Design review of the part shown in the three views and the two pictorial views. Dimensions are in mm from the part's minimum x, y and z. A direction names the side the tool comes from. Coordinates: 2 decimals unless noted, no trailing zeros. Order: outer loops, then holes, each group sorted by start corner. A loop starts at its lowest first (then second) coordinate and runs counter-clockwise, first axis right, second up. Notation, with made-up numbers: (-19.75, 1.5) - (27.25, 1.5) arc R31 cw to (27.25, 30.5) - close; hole circle Ø2 at (64.5, 84). An arc over 180 degrees is marked (long way). One line per item, written item: value. Start each with the question number.
(1) Clearance check with a flat-ended pin moving along its axis: pin 1 (2 mm diameter, centred on x = 5.5, z = 3.5, fed in from -Y). State where the tip first meets the part, or that it passes through.
(2) To check wall thickness, follow line 1 along Z through (x, y) = (0.5, 0.5); line 2 along Y through (x, z) = (5.5, 6.75); line 3 along Z through (x, y) = (4.25, 14). State the ranges of each line that lie inside material, in increasing order.
(3) For the marked faces 1 and 2, list the 3-axis set-ups (+Z, -Z, +X, -X, +Y, -Y) from which the entire face can be reached by the end or side of a thin tool; tool diameter is ignored.
(4) Mouldability with a two-part tool opening along Z and no side actions: class the marked faces 3, 4, 5 and 6 as released by +Z, released by -Z, zero draft, split by the parting line, or undercut.
(5) Consider section A-A on y = 8.25. Write out the cut boundary in (x, z), then the cut area to 3 significant figures.
(6) Consider section C-C on x = 10.75. Write out the cut boundary in (y, z).
(7) Consider section D-D on y = 4. Write out the cut boundary in (x, z).
(8) Consider section B-B on z = 5. Write out the cut boundary in (x, y).
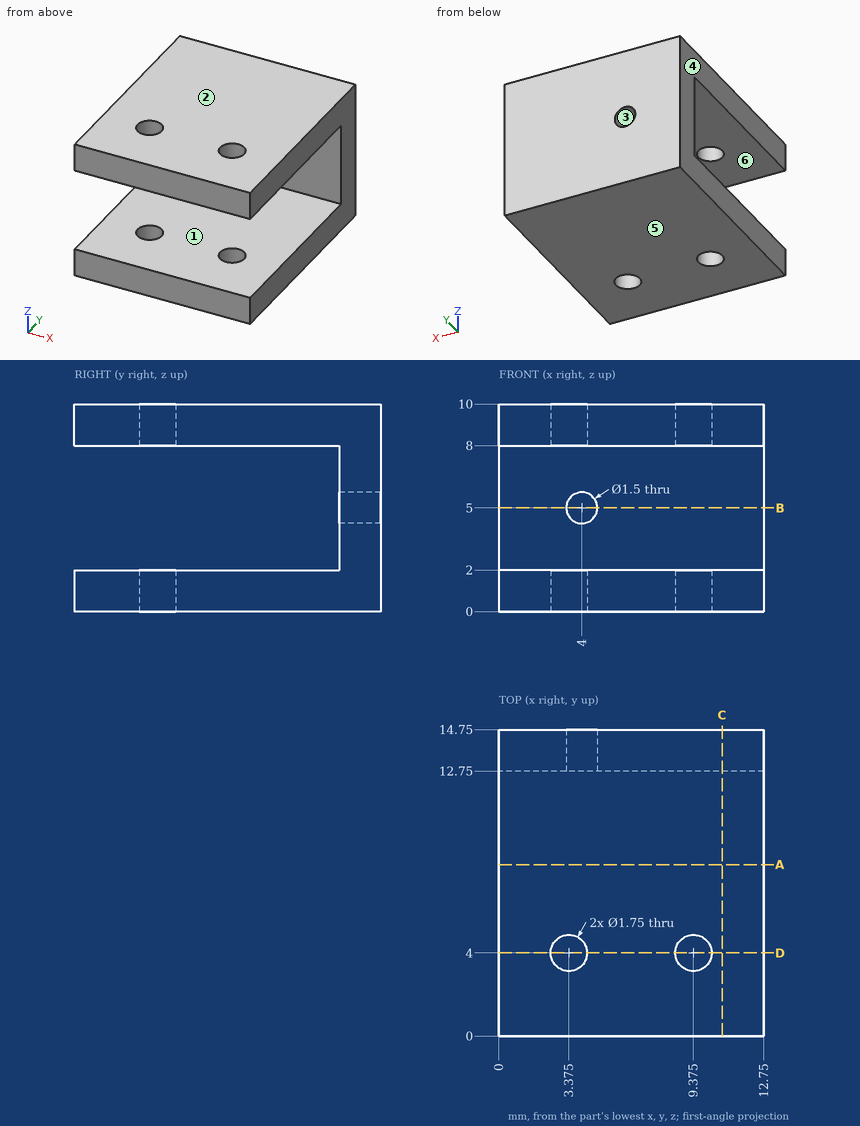
Geometry check:
1. pin 1: stops at y = 12.75
2. line 1: z = 0 to 2, 8 to 10
2. line 2: y = 12.75 to 14.75
2. line 3: z = 0 to 4.29, 5.71 to 10
3. face 1: +X, -X, -Y
3. face 2: +Z, +X, -X, +Y, -Y
4. face 3: undercut
4. face 4: zero draft
4. face 5: released by -Z
4. face 6: undercut
5. outline: (0, 0) - (12.75, 0) - (12.75, 2) - (0, 2) - close; (0, 8) - (12.75, 8) - (12.75, 10) - (0, 10) - close
5. area: 51.0 mm^2
6. outline: (0, 0) - (14.75, 0) - (14.75, 10) - (0, 10) - (0, 8) - (12.75, 8) - (12.75, 2) - (0, 2) - close
7. outline: (0, 0) - (2.5, 0) - (2.5, 2) - (0, 2) - close; (0, 8) - (2.5, 8) - (2.5, 10) - (0, 10) - close; (4.25, 0) - (8.5, 0) - (8.5, 2) - (4.25, 2) - close; (4.25, 8) - (8.5, 8) - (8.5, 10) - (4.25, 10) - close; (10.25, 0) - (12.75, 0) - (12.75, 2) - (10.25, 2) - close; (10.25, 8) - (12.75, 8) - (12.75, 10) - (10.25, 10) - close
8. outline: (0, 12.75) - (3.25, 12.75) - (3.25, 14.75) - (0, 14.75) - close; (4.75, 12.75) - (12.75, 12.75) - (12.75, 14.75) - (4.75, 14.75) - close
